```python
from build123d import *

# Parameters (mm, degrees)
SKETCH3_W          = 14
SKETCH3_H          = 1.5
CHAMFER1_SIZE      = 0.45
CUT_EXTRUDE1_DEPTH = 1.19


with BuildPart() as part:
    # Sketch3 → Revolve1 (revolve)
    with BuildSketch(Plane(origin=(0, 0, 0), x_dir=(0, 0, -1), z_dir=(1, 0, 0))):
        with Locations((0, 0.75)):
            Rectangle(SKETCH3_W, SKETCH3_H)
    revolve(axis=Axis((0, 0, -7), (0, 0, 1)))

    # Chamfer1
    chamfer1_edges = [part.edges().sort_by_distance(p)[0] for p in [
        (0, -1.5, -7),
    ]]
    chamfer(chamfer1_edges, length=CHAMFER1_SIZE)

    # Sketch6 → Revolve2 (revolve)
    with BuildSketch(Plane(origin=(0, 0, 0), x_dir=(0, 0, -1), z_dir=(1, 0, 0))):
        Polygon((-7, 3), (-6.8, 3), (-5.3, 1.5), (-5.3, 0), (-7, 0), align=None)
    revolve(axis=Axis((0, 0, -7), (0, 0, 1)))

    # Sketch8 → Cut-Extrude1 (cut)
    with BuildSketch(Plane.XY.offset(7)):
        Polygon((0, 1.154700538), (-1, 0.577350269), (-1, -0.577350269), (0, -1.154700538), (1, -0.577350269), (1, 0.577350269), align=None)
    extrude(amount=-CUT_EXTRUDE1_DEPTH, mode=Mode.SUBTRACT)

    # Cut-Extrude2 cone 1 section (through the dimple's axis) → Cut-Extrude2 (revolve, cut)
    with BuildSketch(Plane(origin=(0, 0, 7), x_dir=(0, -1, 0), z_dir=(1, 0, 0))):
        Polygon((0, 0), (1.154700538, 0), (0, 1.154700538), align=None)
    revolve(axis=Axis((0, 0, 7), (0, 0, -1)), mode=Mode.SUBTRACT)


solid = part.part
```
Work out the finished part from the listing and answer in its coordinate system (mm). A direction names the side the tool comes from. Coordinates: 2 decimals unless noted, no trailing zeros. Loops run counter-clockwise (first coordinate to the right, second up) from the corner with the lowest first, then second, coordinate; pieces in that order, holes last. Notation, with made-up numbers: (75.25, 11) -> (115.25, 11) arc R15 cw to (115.25, 34) -> close; hole circle Ø10 at (80.5, 34.25). An arc over 180 degrees is marked (long way). Answer as CSV lines item,"result".
Q1. The part is cut by section A-A on y = 0. Write down the section's boundary in (x, z), and give its area (3 significant figures).
Findings:
outline,"(-3, 6.8) -> (-1.5, 5.3) -> (-1.5, -6.55) -> (-1.05, -7) -> (1.05, -7) -> (1.5, -6.55) -> (1.5, 5.3) -> (3, 6.8) -> (3, 7) -> (1.15, 7) -> (1, 6.85) -> (1, 5.81) -> (-1, 5.81) -> (-1, 6.85) -> (-1.15, 7) -> (-3, 7) -> close"
area,"42.2 mm²"
Q2. The part is cut by section B-B on z = 1.25. Write down the section's boundary in (x, y), and give its area (3 significant figures).
Findings:
outline,"circle Ø3 at (0, 0)"
area,"7.07 mm²"
Q3. Find the intervals of material crossed by probe 1 along Z at (x, y) = (0.15, 0.4); probe 2 along X at (y, z) = (0.05, 3.25), in increasing order.
Findings:
probe 1,"z = -7 to 5.81"
probe 2,"x = -1.5 to 1.5"
Q4. Each of these flat-tipped pins is pushed along its axis until it touches: pin 1 (1.5 mm diameter, centred on y = -0.5, z = -5, fed in from -X); pin 2 (3 mm diameter, centred on x = -2.5, y = -2, fed in from -Z); pin 3 (3 mm diameter, centred on x = -2, z = 2.5, fed in from +Y). Where does it stop, or does it pass through?
Findings:
pin 1,"stops at x = -1.5"
pin 2,"stops at z = 5.5"
pin 3,"stops at y = 1.41"
Q5. A tool of negligible diameter and unlimited length cuts with its end or side. For faces 5 (the face through (1, -1, 7)), 6 (the face through (1, 0, 6)), from which of +Z, -Z, +X, -X, +Y, -Y can it reach the whole face along a straight path? Write none if from no direction.
Findings:
face 5,"+Z, +X, -X, +Y, -Y"
face 6,"+Z"
Q6. For a pull along Y with two mould halves and no side action, classify faces 1 (the face through (0.49, -0.87, 6.41)), 2 (the face through (-0.49, 0.87, 6.41)), 3 (the face through (0, 0, -7)), 4 (the face through (-0.07, -1.5, -0.71)) as +Y half, -Y half, draft (parallel to the pull), parting line (faces both ways), or undercut.
Findings:
face 1,"undercut"
face 2,"undercut"
face 3,"draft"
face 4,"parting line"
